from build123d import *

# Parameters (mm, degrees)
F0_W     = 100
F0_H     = 60
F1_DEPTH = 6
F3_DEPTH = 60
F4_R     = 12.5
F5_DEPTH = 1
F6_SIZE  = 15


with BuildPart() as f1:
    # F0 (on Top) → F1 (new body)
    with BuildSketch(Plane.XY):
        Rectangle(F0_W, F0_H)
    extrude(amount=F1_DEPTH)

    # F2 (on face) → F3 (join)
    with BuildSketch(Plane.XY.offset(6)):
        Polygon((44.343146, 30), (-10, -24.343146), (-4.343146, -30), (50, 24.343146), align=None)
    extrude(amount=F3_DEPTH)

    # F4 (on face) → F5 (cut)
    with BuildSketch(Plane(origin=(12.828427, -12.828427, 0), x_dir=(0.707107, 0.707107, 0), z_dir=(0.707107, -0.707107, 0))):
        with Locations((14.142136, 36)):
            Circle(F4_R)
    extrude(amount=-F5_DEPTH, mode=Mode.SUBTRACT)

    # F6
    f6_edges = [f1.edges().sort_by_distance(p)[0] for p in [
        (-7.171573, -27.171573, 66),
        (47.171573, 27.171573, 66),
    ]]
    chamfer(f6_edges, length=F6_SIZE)


solid = f1.part
The listing builds one solid part. Answer for the finished solid, in the listing's coordinates (mm). A direction names the side the tool comes from. Give positions to 0.01 mm unless a question says otherwise; leave off trailing zeros. Order: outer loops, then holes, each group sorted by start corner. A loop starts at its lowest first (then second) coordinate and runs counter-clockwise, first axis right, second up. Notation, with made-up numbers: (59.25, 77) - (96.25, 77) arc R16 cw to (96.25, 83) - close; hole circle Ø5 at (-6, 1). An arc over 180 degrees is marked (long way). Use one line per item in the form item = value.
1) Find section C-C on z = 33. Determine the outline of the cut face in (x, y).
Verdict:
outline = (-10, -24.34) - (-4.34, -30) - (14.25, -11.41) - (13.54, -10.7) - (30.7, 6.46) - (31.41, 5.75) - (50, 24.34) - (44.34, 30) - close
2) Find section B-B on x = -7. Determine the outline of the cut face in (y, z), and give its area (3 significant figures).
Verdict:
outline = (-30, 0) - (30, 0) - (30, 6) - (-21.34, 6) - (-21.34, 55.24) - (-27.34, 51) - (-27.34, 6) - (-30, 6) - close
area = 643 mm^2
3) Find section A-A on y = 17. Determine the outline of the cut face in (x, z), and give its area (3 significant figures).
Verdict:
outline = (-50, 0) - (50, 0) - (50, 6) - (42.66, 6) - (42.66, 61.38) - (36.13, 66) - (31.34, 66) - (31.34, 6) - (-50, 6) - close
area = 1,260 mm^2
4) Consider probe 1 along Z at (x, y) = (-19.5, 14); probe 2 along Y at (x, z) = (6.5, 26); probe 3 along X at (y, z) = (-24, 41). Determine where each line is inside the solid, lowest interval first. Write a range as [from, to].
Verdict:
probe_1 = [0, 6]
probe_2 = [-19.16, -7.84]
probe_3 = [-9.66, 1.66]
5) Each of these flat-tipped pins is pushed along its axis until it touches: pin 1 (10 mm diameter, centred on y = -17.5, z = 17, fed in from +X); pin 2 (10 mm diameter, centred on x = 18, z = 42, fed in from +Y); pin 3 (3 mm diameter, centred on x = 48.5, y = 26, fed in from +Z). Where does it stop, or does it pass through?
Verdict:
pin_1 = 13.16
pin_2 = 8.66
pin_3 = 52.39
6) The mould has two halves that part along X. Classify faces 1 (the flat face through (17.552, 3.209, 35.58)), 2 (the cylindrical face through (20.56, -4.4, 23.8)), 3 (the flat face through (-1, 0, 0)): released by +X, released by -X, zero draft, split by the parting line, or undercut.
Verdict:
face_1 = released by -X
face_2 = undercut
face_3 = zero draft
7) For faces 4 (the flat face through (22.448, -3.209, 22.247)), 5 (the flat face through (48, 28, 6)), 6 (the flat face through (-7.211, -27.132, 28.185)), determine the directions among +Z, -Z, +X, -X, +Y, -Y from which every point of the face is accessible in a straight line to the end or side of a thin tool.
Verdict:
face_4 = +Z, +X, -Y
face_5 = +Z, +X, +Y
face_6 = +Z, -X, -Y
8) Find section D-D on z = 11. Determine the outline of the cut face in (x, y).
Verdict:
outline = (-10, -24.34) - (-4.34, -30) - (50, 24.34) - (44.34, 30) - close
